Geometry: final body of the model. Coordinates: model frame, mm. A direction names the side the tool comes from. Give positions to 0.01 mm unless a question says otherwise; leave off trailing zeros. Write each loop counter-clockwise with the first axis right and the second up, starting at its lowest first coordinate (ties: lowest second). Pieces come first, ordered by that corner, then holes. Notation, with made-up numbers: (21, 22) -> (40, 22) arc R17 cw to (40, 33) -> close; hole circle Ø4 at (-31.5, 26). An arc over 180 degrees is marked (long way). Answer as a JSON object with one key per item and string values.
from build123d import *

# Parameters (mm, degrees)
BOSS_EXTRUDE1_DEPTH   = 6.35
FILLET2_R             = 2.54
FILLET5_SIZE          = 10.16
FILLET5_SIZE_2        = 3.81
FILLET3_R             = 0.762
FILLET4_R             = 1.27
M4X0_7_TAPPED_HOLE1_D = 3.3


with BuildPart() as part:
    # Sketch1 → Boss-Extrude1 (new body)
    with BuildSketch(Plane.XY):
        with BuildLine():
            Line((-49.276, 0.508), (-49.276, 12.192))
            Line((-49.276, 12.192), (-36.576, 12.192))
            ThreePointArc((-36.576, 12.192), (-24.638, 0.254), (-12.7, 12.192))
            Line((-12.7, 12.192), (0, 12.192))
            Line((0, 12.192), (0, 0.508))
            Line((0, 0.508), (3.81, 0.508))
            Line((3.81, 0.508), (3.81, 0))
            Line((3.81, 0), (0, 0))
            Line((0, 0), (0, -5.08))
            Line((0, -5.08), (-1.27, -5.08))
            Line((-1.27, -5.08), (-1.27, 3.302))
            Line((-1.27, 3.302), (-6.985, 3.302))
            Line((-6.985, 3.302), (-6.985, -5.08))
            Line((-6.985, -5.08), (-10.795, -5.08))
            Line((-10.795, -5.08), (-10.795, 0))
            Line((-10.795, 0), (-38.481, 0))
            Line((-38.481, 0), (-38.481, -5.08))
            Line((-38.481, -5.08), (-42.291, -5.08))
            Line((-42.291, -5.08), (-42.291, 3.302))
            Line((-42.291, 3.302), (-48.006, 3.302))
            Line((-48.006, 3.302), (-48.006, -5.08))
            Line((-48.006, -5.08), (-49.276, -5.08))
            Line((-49.276, -5.08), (-49.276, 0))
            Line((-49.276, 0), (-53.086, 0))
            Line((-53.086, 0), (-53.086, 0.508))
            Line((-53.086, 0.508), (-49.276, 0.508))
        make_face()
        with BuildLine():
            Line((-18.478827328, 0.508), (-10.355558408, 0.508))
            Line((-10.355558408, 0.508), (-14.507082252, 3.71758146))
            ThreePointArc((-14.507082252, 3.71758146), (-16.336366742, 1.919018483), (-18.478827328, 0.508))
        make_face(mode=Mode.SUBTRACT)
        with BuildLine():
            Line((-9.525, 1.150112382), (-13.88565937, 4.52137845))
            ThreePointArc((-13.88565937, 4.52137845), (-13.218881773, 5.554605714), (-12.651085576, 6.645366193))
            Line((-12.651085576, 6.645366193), (-9.525, 4.960112382))
            Line((-9.525, 4.960112382), (-9.525, 1.150112382))
        make_face(mode=Mode.SUBTRACT)
        with BuildLine():
            Line((-9.525, 6.738112382), (-12.07736066, 8.107688139))
            ThreePointArc((-12.07736066, 8.107688139), (-11.751952055, 9.293546556), (-11.53824026, 10.504528889))
            Line((-11.53824026, 10.504528889), (-9.525, 9.278112382))
            Line((-9.525, 9.278112382), (-9.525, 6.738112382))
        make_face(mode=Mode.SUBTRACT)
        with BuildLine():
            Line((-39.751, 9.278112382), (-39.751, 6.738112382))
            Line((-39.751, 6.738112382), (-37.19863934, 8.107688139))
            ThreePointArc((-37.19863934, 8.107688139), (-37.524047945, 9.293546556), (-37.73775974, 10.504528889))
            Line((-37.73775974, 10.504528889), (-39.751, 9.278112382))
        make_face(mode=Mode.SUBTRACT)
        with BuildLine():
            Line((-39.751, 4.960112382), (-39.751, 1.150112382))
            Line((-39.751, 1.150112382), (-35.39034063, 4.52137845))
            ThreePointArc((-35.39034063, 4.52137845), (-36.057118227, 5.554605714), (-36.624914424, 6.645366193))
            Line((-36.624914424, 6.645366193), (-39.751, 4.960112382))
        make_face(mode=Mode.SUBTRACT)
        with BuildLine():
            Line((-30.797172672, 0.508), (-38.920441592, 0.508))
            Line((-38.920441592, 0.508), (-34.768917748, 3.71758146))
            ThreePointArc((-34.768917748, 3.71758146), (-32.939633258, 1.919018483), (-30.797172672, 0.508))
        make_face(mode=Mode.SUBTRACT)
    extrude(amount=BOSS_EXTRUDE1_DEPTH)

    # Fillet2
    fillet2_edges = [part.edges().sort_by_distance(p)[0] for p in [
        (-1.27, 3.302, 3.175),
        (-6.985, 3.302, 3.175),
        (-42.291, 3.302, 3.175),
        (-48.006, 3.302, 3.175),
    ]]
    fillet(fillet2_edges, radius=FILLET2_R)

    # Fillet5
    # an asymmetric fillet: 10.16, 3.81 mm, written as the material it adds along each edge
    with BuildSketch(Plane(origin=(0, 0.508, 0), x_dir=(0, 1, 0), z_dir=(0, 0, 1))) as fillet5_piece_1:
        with BuildLine():
            Bezier((FILLET5_SIZE, 0), (0, 0), (0, -FILLET5_SIZE_2), weights=[1, 0.707106781, 1])
            Line((0, -FILLET5_SIZE_2), (0, 0))
            Line((0, 0), (FILLET5_SIZE, 0))
        make_face()
    extrude(amount=6.35)
    with BuildSketch(Plane(origin=(-49.276, 0.508, 0), x_dir=(-1, 0, 0), z_dir=(0, 0, 1))) as fillet5_piece_2:
        with BuildLine():
            Bezier((FILLET5_SIZE_2, 0), (0, 0), (0, -FILLET5_SIZE), weights=[1, 0.707106781, 1])
            Line((0, -FILLET5_SIZE), (0, 0))
            Line((0, 0), (FILLET5_SIZE_2, 0))
        make_face()
    extrude(amount=6.35)

    # Fillet3
    fillet3_edges = [part.edges().sort_by_distance(p)[0] for p in [
        (-9.525, 6.738112382, 3.175),
        (-9.525, 9.278112382, 3.175),
        (-11.53824026, 10.504528889, 3.175),
        (-12.07736066, 8.107688139, 3.175),
        (-36.624914424, 6.645366193, 3.175),
        (-39.751, 4.960112382, 3.175),
        (-35.39034063, 4.52137845, 3.175),
        (-30.797172672, 0.508, 3.175),
        (-34.768917748, 3.71758146, 3.175),
        (-38.920441592, 0.508, 3.175),
        (-14.507082252, 3.71758146, 3.175),
        (-18.478827328, 0.508, 3.175),
        (-10.355558408, 0.508, 3.175),
        (-37.73775974, 10.504528889, 3.175),
        (-39.751, 9.278112382, 3.175),
        (-39.751, 6.738112382, 3.175),
        (-37.19863934, 8.107688139, 3.175),
        (-9.525, 4.960112382, 3.175),
        (-12.651085576, 6.645366193, 3.175),
        (-13.88565937, 4.52137845, 3.175),
    ]]
    fillet(fillet3_edges, radius=FILLET3_R)

    # Fillet4
    fillet4_edges = [part.edges().sort_by_distance(p)[0] for p in [
        (-39.751, 1.150112382, 3.175),
        (-9.525, 1.150112382, 3.175),
    ]]
    fillet(fillet4_edges, radius=FILLET4_R)

    # M4x0.7 Tapped Hole1 (through all)
    with Locations(Plane(origin=(0, 12.192, 0), x_dir=(1, 0, 0), z_dir=(0, 1, 0))):
        with Locations((-4.1275, -3.175)):
            m4x0_7_tapped_hole1 = Hole(M4X0_7_TAPPED_HOLE1_D / 2)

    # Mirror1: M4x0.7 Tapped Hole1 across plane
    add(m4x0_7_tapped_hole1.mirror(Plane(origin=(-24.638, 0, 0), x_dir=(0, 0, 1), z_dir=(1, 0, 0))), mode=Mode.SUBTRACT)


solid = part.part
Q1. Set-up query: faces 4 (the flat face through (-49.276, 11, 3)), 5 (the flat face through (0, -3, 3)), 6 (the flat face through (-26.9, 0.3, 6.35)), 7 (the flat face through (-6.985, -2, 3)), 8 (the cylindrical face through (-14.478, 3.437, 3.219)). Return all of +Z, -Z, +X, -X, +Y, -Y with unobstructed straight access to the full face (end or side cutting, diameter ignored); none if empty.
Values:
{"face 4": "+Z, -Z, -X, +Y", "face 5": "+Z, -Z, +X, -Y", "face 6": "+Z, +X, -X, +Y, -Y", "face 7": "+Z, -Z, -Y", "face 8": "+Z, -Z"}
Q2. Cut plane A-A (x = -3). Return the cut outline in (y, z), and give its area (3 significant figures).
Values:
{"outline": "(3.17, 0) -> (12.19, 0) -> (12.19, 1.97) -> (3.17, 1.97) -> close; (3.17, 4.38) -> (12.19, 4.38) -> (12.19, 6.35) -> (3.17, 6.35) -> close", "area": "35.6 mm²"}
Q3. Material intervals for L1, parallel to X at y = -3.5, z = 2.5 (3 decimals); L2, parallel to Y at x = -11.5, z = 2.5; L3, parallel to X at y = 1.75, z = 1.5, sorted ascending. Write a range as from..to.
Values:
{"L1": "-49.276..-48.006, -42.291..-38.481, -10.795..-6.985, -1.27..0", "L2": "0..2.68, 6.02..7.8, 9.82..12.19", "L3": "-51.26..-47.81, -42.49..-37.28, -32.76..-30.42, -18.85..-16.52, -12..-6.78, -1.47..1.98"}
Q4. First-contact query: P1, Ø3, axis at x = -24, z = 5, coming from the +Y side; P2, Ø0.7, axis at x = -45.5, z = 1, coming from the -Y side; P3, Ø0.9, axis at y = 8.5, z = 4, coming from the -X side. Flat tips, straight axial feed; report the tip coordinate or a pass-through.
Values:
{"P1": "y = 0.45", "P2": "y = 3.27", "P3": "x = -49.4"}
Q5. Cut plane C-C (z = 3.75). State how many separate pieces and enclosed holes the cut face has, and give its area (3 significant figures).
Values:
{"separate pieces": "3", "enclosed holes": "6", "area": "309 mm²"}
Q6. Mould query, pull axis Y, two halves, no side actions, for faces 1 (the flat face through (0, 11, 3)), 2 (the flat face through (-6, 12.192, 3)), 3 (the cylindrical face through (-9.91, 7.35, 3.22)). Classes: pulls with the +Y half, pulls with the -Y half, needs draft (parallel to the pull), parting line crosses it, or undercut.
Values:
{"face 1": "needs draft", "face 2": "pulls with the +Y half", "face 3": "undercut"}
Q7. Cut plane D-D (x = -44). Return the cut outline in (y, z).
Values:
{"outline": "(3.16, 0) -> (12.19, 0) -> (12.19, 1.99) -> (3.16, 1.99) -> close; (3.16, 4.36) -> (12.19, 4.36) -> (12.19, 6.35) -> (3.16, 6.35) -> close"}
Q8. Cut plane B-B (y = -2.25). Return the cut outline in (x, z) (3 decimals).
Values:
{"outline": "(-49.276, 0) -> (-48.006, 0) -> (-48.006, 6.35) -> (-49.276, 6.35) -> close; (-42.291, 0) -> (-38.481, 0) -> (-38.481, 6.35) -> (-42.291, 6.35) -> close; (-10.795, 0) -> (-6.985, 0) -> (-6.985, 6.35) -> (-10.795, 6.35) -> close; (-1.27, 0) -> (0, 0) -> (0, 6.35) -> (-1.27, 6.35) -> close"}
